Geometry: final body of the model. Coordinates: model frame, mm. A direction names the side the tool comes from. Coordinates: 2 decimals unless noted, no trailing zeros. Write each loop counter-clockwise with the first axis right and the second up, starting at its lowest first coordinate (ties: lowest second). Pieces come first, ordered by that corner, then holes. Notation, with made-up numbers: M 78,17 L 90,17 A22 cw 90,42 Z; hole C 61,49.5 d6. An arc over 180 degrees is marked long. Write item = value, one per line. Start each with the question number.
Item 1: First-contact query: pin 1 Ø1.7 at (x, z) = (22.5, -19) entering from +Y; pin 2 Ø2.5 at (y, z) = (16.5, -28) entering from -X; pin 3 Ø1.5 at (y, z) = (16, -28) entering from -X. Flat tips, straight axial feed; report the tip coordinate or a pass-through.
Item 2: Section A-A on z = 12. Output: boundary loops of the cut face in (x, y) (1 decimal).
Item 3: Section C-C on y = 15. Output: boundary loops of the cut face in (x, z) (3 decimals), plus the area to 3 significant figures.
Item 4: Ray query, L1, parallel to X at y = 8, z = -19 (3 decimals); L2, parallel to Z at x = -23.5, y = 36.5; L3, parallel to X at y = 13, z = -16.5 (3 decimals). Return the intervals inside material, ascending. Write a range as [from, to].
Item 5: Reachability of faces 4 (the flat face through (-15, 13.03, -28)), 5 (the cylindrical face through (-33.079, 32.452, 28.576)), 6 (the flat face through (0, 35, 25)), 7 (the cylindrical face through (-24.55, 8.211, -16.507)), 8 (the cylindrical face through (33.001, 32.452, 28.654)) from +Z, -Z, +X, -X, +Y, -Y: full face, straight path, thin tool, end or side. Return the list, or none.
Item 6: Pull-direction query (X, two-part tool) for faces 1 (the flat face through (29, 57.658, 25)), 2 (the flat face through (-34.505, 32, 0)), 3 (the flat face through (34.505, 32, 0)); classes: +X half, -X half, draft (parallel to the pull), parting line (faces both ways), or undercut.
Item 7: Section B-B on y = 27. Output: boundary loops of the cut face in (x, z) (3 decimals).
Item 8: Section D-D on z = -12. Give the number of separate pieces and of enclosed holes in the cut face, plus the area to 3 significant figures.
from build123d import *

# Parameters (mm, degrees)
SKETCH1_W                  = 69.01
SKETCH1_H                  = 60.16
BOSS_EXTRUDE3_DEPTH        = 64.008
SKETCH2_W                  = 58.85
SKETCH2_H                  = 50
CUT_EXTRUDE4_DEPTH         = 58.928
FILLET1_R                  = 5
SKETCH3_R                  = 4.8067
BOSS_EXTRUDE4_DEPTH        = 11.43
SKETCH3_3_R                = 2.8067
CUT_EXTRUDE5_DEPTH         = 6.35
SKETCH9_R                  = 4.8067
SKETCH9_R_2                = 2.8067
BOSS_EXTRUDE5_DEPTH        = 6.35
SKETCH10_R                 = 2.159
CUT_EXTRUDE6_DEPTH         = 5.08
BOSS_EXTRUDE6_DEPTH        = 1
FACE_2_CONNECTOR_HOLES_W   = 6.4
FACE_2_CONNECTOR_HOLES_H   = 5
FACE_2_CONNECTOR_HOLES_W_2 = 10.4
CUT_EXTRUDE7_DEPTH         = 5.08
FACE_3_CONNECTOR_HOLES_W   = 6.4
FACE_3_CONNECTOR_HOLES_H   = 5
CUT_EXTRUDE8_DEPTH         = 5.08


with BuildPart() as part:
    # Sketch1 → Boss-Extrude3 (new body)
    with BuildSketch(Plane(origin=(0, 0, 0), x_dir=(1, 0, 0), z_dir=(0, 1, 0))):
        Rectangle(SKETCH1_W, SKETCH1_H)
    extrude(amount=BOSS_EXTRUDE3_DEPTH)

    # Sketch2 → Cut-Extrude4 (cut)
    with BuildSketch(Plane(origin=(0, 64.008, 0), x_dir=(1, 0, 0), z_dir=(0, 1, 0))):
        Rectangle(SKETCH2_W, SKETCH2_H)
    extrude(amount=-CUT_EXTRUDE4_DEPTH, mode=Mode.SUBTRACT)

    # Fillet1
    fillet1_edges = [part.edges().sort_by_distance(p)[0] for p in [
        (-34.505, 32.004, 30.08),
        (34.505, 32.004, 30.08),
        (34.505, 32.004, -30.08),
        (-34.505, 32.004, -30.08),
    ]]
    fillet(fillet1_edges, radius=FILLET1_R)

    # Sketch3 → Boss-Extrude4 (add)
    with BuildSketch(Plane(origin=(0, 64.008, 0), x_dir=(1, 0, 0), z_dir=(0, 1, 0))):
        with Locations((-29.425, 25)):
            Circle(SKETCH3_R)
        with Locations((29.425, 25)):
            Circle(SKETCH3_R)
        with Locations((-29.425, -25)):
            Circle(SKETCH3_R)
        with Locations((29.425, -25)):
            Circle(SKETCH3_R)
    extrude(amount=-BOSS_EXTRUDE4_DEPTH)

    # Sketch3<3> → Cut-Extrude5 (cut)
    with BuildSketch(Plane(origin=(0, 64.008, 0), x_dir=(1, 0, 0), z_dir=(0, 1, 0))):
        with Locations(Location((-29.425, 25, 0), (0, 0, 270))):
            Circle(SKETCH3_3_R)
        with Locations(Location((29.425, 25, 0), (0, 0, 270))):
            Circle(SKETCH3_3_R)
        with Locations(Location((29.425, -25, 0), (0, 0, 270))):
            Circle(SKETCH3_3_R)
        with Locations(Location((-29.425, -25, 0), (0, 0, 270))):
            Circle(SKETCH3_3_R)
    extrude(amount=-CUT_EXTRUDE5_DEPTH, mode=Mode.SUBTRACT)

    # Sketch9 → Boss-Extrude5 (add)
    # profile 1 of 4: a face of its own
    with BuildSketch(Plane(origin=(0, 5.08, 0), x_dir=(1, 0, 0), z_dir=(0, 1, 0))):
        with Locations(Location((-23.475, 19.1, 0), (0, 0, 90))):
            Circle(SKETCH9_R)
        with Locations(Location((-23.475, 19.1, 0), (0, 0, 270))):
            Circle(SKETCH9_R_2, mode=Mode.SUBTRACT)
    # profile 2 of 4: a face of its own
    with BuildSketch(Plane(origin=(0, 5.08, 0), x_dir=(1, 0, 0), z_dir=(0, 1, 0))):
        with Locations(Location((23.275, 19.1, 0), (0, 0, 90))):
            Circle(SKETCH9_R)
        with Locations(Location((23.275, 19.1, 0), (0, 0, 270))):
            Circle(SKETCH9_R_2, mode=Mode.SUBTRACT)
    # profile 3 of 4: a face of its own
    with BuildSketch(Plane(origin=(0, 5.08, 0), x_dir=(1, 0, 0), z_dir=(0, 1, 0))):
        with Locations(Location((23.275, -18.9, 0), (0, 0, 90))):
            Circle(SKETCH9_R)
        with Locations(Location((23.275, -18.9, 0), (0, 0, 270))):
            Circle(SKETCH9_R_2, mode=Mode.SUBTRACT)
    # profile 4 of 4: a face of its own
    with BuildSketch(Plane(origin=(0, 5.08, 0), x_dir=(1, 0, 0), z_dir=(0, 1, 0))):
        with Locations(Location((-23.475, -19.15, 0), (0, 0, 90))):
            Circle(SKETCH9_R)
        with Locations(Location((-23.475, -19.15, 0), (0, 0, 270))):
            Circle(SKETCH9_R_2, mode=Mode.SUBTRACT)
    extrude(amount=BOSS_EXTRUDE5_DEPTH)

    # Sketch10 → Cut-Extrude6 (cut)
    with BuildSketch(Plane(origin=(0, 5.08, 0), x_dir=(1, 0, 0), z_dir=(0, 1, 0))):
        with Locations(Location((14.2125, 12, 0), (0, 0, 270))):
            Circle(SKETCH10_R)
        with Locations(Location((14.2125, -12, 0), (0, 0, 270))):
            Circle(SKETCH10_R)
        with Locations(Location((-14.2125, 12, 0), (0, 0, 270))):
            Circle(SKETCH10_R)
        with Locations(Location((-14.2125, -12, 0), (0, 0, 270))):
            Circle(SKETCH10_R)
    extrude(amount=-CUT_EXTRUDE6_DEPTH, mode=Mode.SUBTRACT)

    # Sketch12 → Boss-Extrude6 (add)
    with BuildSketch(Plane(origin=(0, 5.08, 0), x_dir=(1, 0, 0), z_dir=(0, 1, 0))):
        Polygon((-26.546494391, 13.413188801), (-25.899358974, 13.413188801), (-25.899358974, 9.913188801), (-26.213461538, 9.913188801), (-26.213461538, 13.054214442), (-26.751923077, 13.054214442), align=None)
    extrude(amount=BOSS_EXTRUDE6_DEPTH)

    # Face 2 Connector Holes → Cut-Extrude7 (cut)
    with BuildSketch(Plane(origin=(0, 0, -30.08), x_dir=(-1, 0, 0), z_dir=(0, 0, -1))):
        with Locations((15.305, 15.53)):
            Rectangle(FACE_2_CONNECTOR_HOLES_W, FACE_2_CONNECTOR_HOLES_H)
        with Locations((-13.045, 15.53)):
            Rectangle(FACE_2_CONNECTOR_HOLES_W_2, FACE_2_CONNECTOR_HOLES_H)
    extrude(amount=-CUT_EXTRUDE7_DEPTH, mode=Mode.SUBTRACT)

    # Face 3 Connector Holes → Cut-Extrude8 (cut)
    with BuildSketch(Plane(origin=(34.505, 0, 0), x_dir=(0, 0, -1), z_dir=(1, 0, 0))):
        with Locations((9.93, 15.53)):
            Rectangle(FACE_3_CONNECTOR_HOLES_W, FACE_3_CONNECTOR_HOLES_H)
    extrude(amount=-CUT_EXTRUDE8_DEPTH, mode=Mode.SUBTRACT)


solid = part.part
Responses:
q1.pin_1 = 5.08
q1.pin_2 = -34.22
q1.pin_3 = -34.01
q2.outline = M -34.5,0 L -16.4,0 L -16.4,5.1 L -29.4,5.1 L -29.4,64 L -34.5,64 Z; M -12.1,0 L 12.1,0 L 12.1,5.1 L -12.1,5.1 Z; M 16.4,0 L 34.5,0 L 34.5,64 L 29.4,64 L 29.4,5.1 L 16.4,5.1 Z
q3.outline = M -34.505,-25.08 A5 ccw -29.505,-30.08 L -18.505,-30.08 L -18.505,-25 L -29.425,-25 L -29.425,25 L 29.425,25 L 29.425,-6.73 L 34.505,-6.73 L 34.505,25.08 A5 ccw 29.505,30.08 L -29.505,30.08 A5 ccw -34.505,25.08 Z; M -12.105,-30.08 L 7.845,-30.08 L 7.845,-25 L -12.105,-25 Z; M 18.245,-30.08 L 29.505,-30.08 A5 ccw 34.505,-25.08 L 34.505,-13.13 L 29.425,-13.13 L 29.425,-25 L 18.245,-25 Z
q3.area = 1,070 mm²
q4.L1 = [-34.505, -29.425], [-28.281, -26.28], [-20.67, -18.669], [18.469, 20.47], [26.08, 28.081], [29.425, 34.505]
q4.L2 = [-30.08, -25], [25, 30.08]
q4.L3 = [-34.505, -29.425], [29.425, 34.505]
q5.face_4 = -Z
q5.face_5 = +Z, -X, +Y, -Y
q5.face_6 = none
q5.face_7 = +Y
q5.face_8 = +Z, +X, +Y, -Y
q6.face_1 = undercut
q6.face_2 = -X half
q6.face_3 = +X half
q7.outline = M -34.505,-25.08 A5 ccw -29.505,-30.08 L 29.505,-30.08 A5 ccw 34.505,-25.08 L 34.505,25.08 A5 ccw 29.505,30.08 L -29.505,30.08 A5 ccw -34.505,25.08 Z; hole M -29.425,-25 L 29.425,-25 L 29.425,25 L -29.425,25 Z
q8.separate_pieces = 4
q8.enclosed_holes = 0
q8.area = 880 mm²
